The model under review builds one solid part; all positions refer to its coordinate system, in mm. Coordinates: 2 decimals unless noted, no trailing zeros. Loops run counter-clockwise (first coordinate to the right, second up) from the corner with the lowest first, then second, coordinate; pieces in that order, holes last. Notation, with made-up numbers: M 82.5,44.5 L 112.5,44.5 A6 cw 112.5,51.5 Z; hole C 6,40.25 d10. An arc over 180 degrees is marked long. Use CSV: the item, a comma, the result in double quotes. Start each with the question number.
1. Add section C-C, the plane x = 113.5. Write out the cut boundary in (y, z) (3 decimals), then the cut area to 3 significant figures.
2. Clearance check with flat-ended pins moving along their axes: P1, Ø1.6, axis at x = 165.5, z = 2, coming from the +Y side; P2, Ø1.6, axis at y = 71.5, z = 1, coming from the +X side; P3, Ø1, axis at y = 58, z = 1, coming from the -X side. State where each tip first meets the part, or that it passes through.
3. Add section A-A, the plane x = 64.5. Write out the cut boundary in (y, z) (3 decimals), then the cut area to 3 significant figures.
4. Add section D-D, the plane x = 168.5. Write out the cut boundary in (y, z) (3 decimals).
5. For L1, parallel to X at y = 74.5, z = 1.7; L2, parallel to Y at x = 166, z = 1.65; L3, parallel to Y at x = 97, z = 1.4, list the stretches that pass through material, from the lowest coordinate up.
6. Add section B-B, the plane z = 2.1. State how many separate pieces and enclosed holes the cut face has, then the cut area to 3 significant figures.
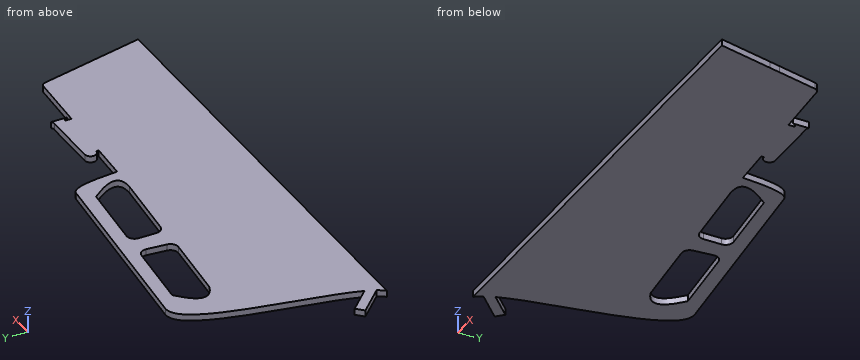
from build123d import *

# Parameters (mm, degrees)
BOSS_EXTRUDE1_DEPTH = 3.175
CUT_EXTRUDE1_DEPTH  = 3.175


with BuildPart() as part:
    # Sketch1 → Boss-Extrude1 (new body)
    with BuildSketch(Plane.XY):
        with BuildLine():
            add(Edge.make_bspline(
                [(2.579059818, 3.776412267), (1.767727302, 2.156821837), (0.911850586, 0.875503614), (0, 0)],
                knots=[0.923802309, 0.923802309, 0.923802309, 0.923802309, 1, 1, 1, 1], degree=3))
            Line((0, 0), (228.6, 0))
            Line((228.6, 0), (222.76882451, 26.801768915))
            Line((222.76882451, 26.801768915), (221.564922434, 32.335251021))
            Line((221.564922434, 32.335251021), (217.266059518, 52.094068206))
            ThreePointArc((217.266059518, 52.094068206), (216.431616334, 53.487306889), (214.923678652, 54.090244201))
            Line((214.923678652, 54.090244201), (186.335881614, 55.663335735))
            Line((186.335881614, 55.663335735), (186.335881614, 58.711335735))
            ThreePointArc((186.335881614, 58.711335735), (186.392581362, 58.712200587), (186.449281111, 58.711335735))
            ThreePointArc((186.449281111, 58.711335735), (187.700530121, 58.174263199), (188.250106948, 56.928455707))
            Line((188.250106948, 56.928455707), (188.250106948, 64.751418591))
            ThreePointArc((188.250106948, 64.751418591), (187.302878972, 64.075530467), (186.139401367, 64.095163563))
            Line((186.139401367, 64.095163563), (158.379745694, 64.095163563))
            ThreePointArc((158.379745694, 64.095163563), (155.621285283, 61.22392358), (158.492525265, 58.46546317))
            Line((158.492525265, 58.46546317), (158.492525265, 57.19546317))
            Line((158.492525265, 57.19546317), (139.704230031, 58.229320662))
            add(Edge.make_bspline(
                [(139.704230031, 58.229320662), (139.045260228, 67.775421627), (137.97702794, 82.099142771), (132.841802065, 82.099142771)],
                knots=[0, 0, 0, 0, 1, 1, 1, 1], degree=3))
            Line((132.841802065, 82.099142771), (33.135927245, 91.696329699))
            add(Edge.make_bspline(
                [(33.135927245, 91.696329699), (29.992946755, 91.696329699), (16.218901468, 82.07109656), (11.469233026, 28.631681198), (4.58927934, 8.68731164)],
                knots=[0, 0, 0, 0, 0.15232143, 0.857980154, 0.857980154, 0.857980154, 0.857980154], degree=3))
            Line((4.58927934, 8.68731164), (-5.906819212, 19.183410193))
            Line((-5.906819212, 19.183410193), (-9.36737866, 15.722850745))
            Line((-9.36737866, 15.722850745), (2.579059818, 3.776412267))
        make_face()
    extrude(amount=BOSS_EXTRUDE1_DEPTH)

    # Sketch2 → Cut-Extrude1 (cut)
    with BuildSketch(Plane.XY.offset(3.175)):
        with BuildLine():
            Line((41.317655172, 83.967201614), (75.625183332, 80.664931197))
            ThreePointArc((75.625183332, 80.664931197), (78.199946888, 79.296016613), (79.052610873, 76.507415058))
            Line((79.052610873, 76.507415058), (78.107945762, 66.693220334))
            ThreePointArc((78.107945762, 66.693220334), (76.739031178, 64.118456778), (73.950429623, 63.265792793))
            Line((73.950429623, 63.265792793), (39.642901463, 66.568063209))
            add(Edge.make_bspline(
                [(41.317655172, 83.967201614), (25.947965106, 71.264134292), (39.642901463, 66.568063209)],
                knots=[0, 0, 0, 1, 1, 1], degree=2))
        make_face()
        with BuildLine():
            Line((92.508115474, 79.039864911), (126.433071175, 75.774418999))
            add(Edge.make_bspline(
                [(126.433071175, 75.774418999), (140.857755692, 58.596738855), (126.433071175, 59.233433778)],
                knots=[0, 0, 0, 1, 1, 1], degree=2))
            Line((126.433071175, 59.233433778), (91.778026876, 62.569154354))
            ThreePointArc((91.778026876, 62.569154354), (89.322883346, 63.799861058), (88.333071175, 66.361626194))
            Line((88.333071175, 66.361626194), (88.333071175, 75.247393071))
            ThreePointArc((88.333071175, 75.247393071), (89.581306039, 78.0675809), (92.508115474, 79.039864911))
        make_face()
    extrude(amount=-CUT_EXTRUDE1_DEPTH, mode=Mode.SUBTRACT)


solid = part.part
Computed:
1,outline,"M 0,0 L 60.478,0 L 60.478,3.175 L 0,3.175 Z; M 77.019,0 L 83.961,0 L 83.961,3.175 L 77.019,3.175 Z"
1,area,"214 mm^2"
2,P1,"stops at y = 64.1"
2,P2,"stops at x = 138.49"
2,P3,"stops at x = 15.41"
3,outline,"M 0,0 L 64.175,0 L 64.175,3.175 L 0,3.175 Z; M 81.736,0 L 88.677,0 L 88.677,3.175 L 81.736,3.175 Z"
3,area,"226 mm^2"
4,outline,"M 0,0 L 64.095,0 L 64.095,3.175 L 0,3.175 Z"
5,L1,"x = 19.82 to 33.47, 78.86 to 88.33, 127.48 to 137.79"
5,L2,"y = 0 to 64.1"
5,L3,"y = 0 to 62.07, 78.61 to 85.55"
6,separate pieces,"1"
6,enclosed holes,"2"
6,area,"14,500 mm^2"
